Autodesk Inventor part; units mm, degrees
ref_plane "YZ Plane" through (0, 0, 0) normal (1, 0, 0) x (0, 1, 0)
ref_plane "XZ Plane" through (0, 0, 0) normal (0, 1, 0) x (-1, 0, 0)
ref_plane "XY Plane" through (0, 0, 0) normal (0, 0, 1) x (1, 0, 0)
sketch "Skizze1" plane through (0, 0, 0) normal (0, 0, 1) x (1, 0, 0)
  line L0 (-99.7629, 0) -> (488.2371, 0)
  line L1 (0, -39.9766) -> (0, 128.0234)
  line L2 (-5.7629, 94.0234) -> (394.2371, 94.0234)
  line L3 (394.2371, 94.0234) -> (394.2371, -5.9766)
  line L4 (394.2371, -5.9766) -> (-5.7629, -5.9766)
  line L5 (-5.7629, -5.9766) -> (-5.7629, 94.0234)
  line L6 (80.2371, 94.0234) -> (80.2371, -5.9766)
  line L7 (83.2371, -5.9766) -> (83.2371, 94.0234)
  line L8 (169.2371, 94.0234) -> (169.2371, -5.9766)
  line L9 (172.2371, -5.9766) -> (172.2371, 94.0234)
  line L10 (258.2371, 94.0234) -> (258.2371, -5.9766)
  line L11 (268.2371, -5.9766) -> (268.2371, 94.0234)
  line L12 (-15.7629, 104.0234) -> (404.2371, 104.0234)
  line L13 (404.2371, 104.0234) -> (404.2371, -15.9766)
  line L14 (404.2371, -15.9766) -> (-15.7629, -15.9766)
  line L15 (-15.7629, -15.9766) -> (-15.7629, 104.0234)
  point P0 (0, 0)
  point P1 (274.2371, 94.0234)
  point P2 (180.9371, 94.0234)
  point P3 (87.6371, 94.0234)
  dimension "d0" = 100
  dimension "d1" = 400
  dimension "d2" = 120
  dimension "d11" = 10
  dimension "d12" = 10
  dimension "d13" = 10
  dimension "d14" = 10
  dimension "d20" = 86
  dimension "d21" = 86
  dimension "d22" = 86
  dimension "d23" = 3
  dimension "d24" = 3
  dimension "d25" = 10
extrude "Extrusion1" add sketch "Skizze1" along normal blind 150 contours L15 L12 L1 L2 L5 L0 | L0 L5 L4 L1 L14 L15 | L1 L4 L3 L0 L13 L14 | L12 L13 L0 L3 L2 L1 | L6 L2 L7 L0 | L0 L7 L4 L6 | L8 L2 L9 L0 | L0 L9 L4 L8 | L11 L4 L10 L0 | L0 L10 L2 L11
sketch "Skizze2" plane through (0, 0, 0) normal (0, 0, -1) x (-1, 0, 0)
  line L0 (15.7629, -15.9766) -> (-404.2371, -15.9766)
  line L1 (-404.2371, -15.9766) -> (-404.2371, 104.0234)
  line L2 (15.7629, -15.9766) -> (-404.2371, -15.9766)
  line L3 (-404.2371, -15.9766) -> (-404.2371, 104.0234)
  line L4 (-404.2371, 104.0234) -> (15.7629, 104.0234)
  line L5 (15.7629, 104.0234) -> (15.7629, -15.9766)
  point P0 (0, 0)
extrude "Extrusion2" add sketch "Skizze2" along normal blind 10
sketch "Skizze3" plane through (80.2371, -5.9766, 150) normal (-1, 0, 0) x (0, 0, 1)
  point P0 (-150, 5.9766)
sketch "Skizze4" plane through (0, 0, 150) normal (0, 0, 1) x (1, 0, 0)
  line L0 (-13.2629, 101.5234) -> (265.7371, 101.5234)
  line L1 (265.7371, 101.5234) -> (265.7371, 96.5234)
  line L2 (265.7371, 96.5234) -> (-13.2629, 96.5234)
  line L3 (-13.2629, 96.5234) -> (-13.2629, 101.5234)
  line L4 (260.7371, 96.5234) -> (265.7371, 96.5234)
  line L5 (265.7371, 96.5234) -> (265.7371, -13.6946)
  line L6 (265.7371, -13.6946) -> (260.7371, -13.6946)
  line L7 (260.7371, -13.6946) -> (260.7371, 96.5234)
  line L8 (260.7371, -8.4766) -> (-13.2629, -8.4766)
  line L9 (-13.2629, -8.4766) -> (-13.2629, -13.4766)
  line L10 (-13.2629, -13.4766) -> (260.7371, -13.4766)
  line L11 (260.7371, -13.4766) -> (260.7371, -8.4766)
  line L12 (-13.2629, -8.4766) -> (-8.2629, -8.4766)
  line L13 (-8.2629, -8.4766) -> (-8.2629, 96.5234)
  line L14 (-8.2629, 96.5234) -> (-13.2629, 96.5234)
  line L15 (-13.2629, 96.5234) -> (-13.2629, -8.4766)
  line L16 (404.2371, 104.0234) -> (-15.7629, 104.0234)
  line L17 (-5.7629, 94.0234) -> (80.2371, 94.0234)
  line L18 (-5.7629, -5.9766) -> (-5.7629, 94.0234)
  line L19 (-15.7629, 104.0234) -> (-15.7629, -15.9766)
  line L20 (80.2371, -5.9766) -> (-5.7629, -5.9766)
  line L21 (-15.7629, -15.9766) -> (404.2371, -15.9766)
  line L22 (258.2371, 94.0234) -> (258.2371, -5.9766)
  line L23 (268.2371, -5.9766) -> (268.2371, 94.0234)
  point P0 (0, 0)
  point P1 (400.2371, 104.0234)
  point P2 (-11.7629, 104.0234)
  point P3 (-15.7629, 100.0234)
  point P4 (-15.7629, -11.9766)
  point P5 (-11.7629, -15.9766)
  point P6 (400.2371, -15.9766)
  point P7 (-13.2629, 96.5234)
  dimension "d26" = 2.5
  dimension "d27" = 2.5
  dimension "d28" = 2.5
  dimension "d29" = 2.5
  dimension "d30" = 2.5
  dimension "d31" = 2.5
  dimension "d32" = 2.5
  dimension "d33" = 2.5
  dimension "d34" = 2.5
extrude "Extrusion3" cut sketch "Skizze4" against normal blind 5 contours L0 L1 L2 L3 | L2 L13 L8 L15 | L5 L6 L7 L2 | L8 L7 L10 L9
properties part number "3Eier_größer" material "Acetalharz, Schwarz"
For this review, take the finished solid that the model builds, in its own axes (mm). A direction names the side the tool comes from. Round coordinates to 2 decimals unless told otherwise and drop trailing zeros. Write each loop counter-clockwise with the first axis right and the second up, starting at its lowest first coordinate (ties: lowest second). Pieces come first, ordered by that corner, then holes. Notation, with made-up numbers: (-35, 18) - (1, 18) arc R19 cw to (1, 55) - close; hole circle Ø5 at (43, -2). An arc over 180 degrees is marked (long way). Put each result on its own line as item: value.
Q1. We need section A-A (x = 249.5). Give the boundary of the cut face in (y, z).
Solved:
outline: (-15.98, -10) - (104.02, -10) - (104.02, 150) - (101.52, 150) - (101.52, 145) - (96.52, 145) - (96.52, 150) - (94.02, 150) - (94.02, 0) - (-5.98, 0) - (-5.98, 150) - (-8.48, 150) - (-8.48, 145) - (-13.48, 145) - (-13.48, 150) - (-15.98, 150) - close
Q2. Insertion check: pin 1 Ø6 at (x, y) = (50.5, 6) entering from +Z. The pin has a flat end and moves straight along its axis. Give the tip position at first contact, or say it passes through.
Solved:
pin 1: stops at z = 0
Q3. Wall thickness on probe 1 along X at (y, z) = (-5.5, 69); probe 2 along Y at (x, z) = (42.5, 66.5); probe 3 along Z at (x, y) = (255, 46.5): over which ranges is each line inside the solid? List them lowest first.
Solved:
probe 1: x = -15.76 to -5.76, 80.24 to 83.24, 169.24 to 172.24, 258.24 to 268.24, 394.24 to 404.24
probe 2: y = -15.98 to -5.98, 94.02 to 104.02
probe 3: z = -10 to 0
Q4. Mouldability with a two-part tool opening along X and no side actions: class faces 3 (the face through (169.237, 45, 74)), 4 (the face through (-15.763, 45, 71)), 5 (the face through (191, -15.977, 71)) as released by +X, released by -X, zero draft, split by the parting line, or undercut.
Solved:
face 3: undercut
face 4: released by -X
face 5: zero draft
Q5. Machinability: for faces 1 (the face through (268.237, 43, 74)), 2 (the face through (197, 45, -10)), which of the approach directions +Z, -Z, +X, -X, +Y, -Y give a long, thin tool a straight path to every point of the face, cutting with its end or side? Answer none if there is none.
Solved:
face 1: +Z
face 2: -Z, +X, -X, +Y, -Y
Q6. We need section B-B (z = 86). Give the boundary of the cut face in (x, y), and give its area (3 significant figures).
Solved:
outline: (-15.76, -15.98) - (404.24, -15.98) - (404.24, 104.02) - (-15.76, 104.02) - close; hole (-5.76, -5.98) - (80.24, -5.98) - (80.24, 94.02) - (-5.76, 94.02) - close; hole (83.24, -5.98) - (169.24, -5.98) - (169.24, 94.02) - (83.24, 94.02) - close; hole (172.24, -5.98) - (258.24, -5.98) - (258.24, 94.02) - (172.24, 94.02) - close; hole (268.24, -5.98) - (394.24, -5.98) - (394.24, 94.02) - (268.24, 94.02) - close
area: 12,000 mm2
Q7. We need section D-D (x = 292). Give the boundary of the cut face in (y, z).
Solved:
outline: (-15.98, -10) - (104.02, -10) - (104.02, 150) - (94.02, 150) - (94.02, 0) - (-5.98, 0) - (-5.98, 150) - (-15.98, 150) - close
Q8. We need section C-C (y = 86.5). Give the boundary of the cut face in (x, z).
Solved:
outline: (-15.76, -10) - (404.24, -10) - (404.24, 150) - (394.24, 150) - (394.24, 0) - (268.24, 0) - (268.24, 150) - (265.74, 150) - (265.74, 145) - (260.74, 145) - (260.74, 150) - (258.24, 150) - (258.24, 0) - (172.24, 0) - (172.24, 150) - (169.24, 150) - (169.24, 0) - (83.24, 0) - (83.24, 150) - (80.24, 150) - (80.24, 0) - (-5.76, 0) - (-5.76, 150) - (-8.26, 150) - (-8.26, 145) - (-13.26, 145) - (-13.26, 150) - (-15.76, 150) - close
